Geometry: final body of the model. Coordinates: model frame, mm. A direction names the side the tool comes from. Round coordinates to 2 decimals unless told otherwise and drop trailing zeros. Loops run counter-clockwise (first coordinate to the right, second up) from the corner with the lowest first, then second, coordinate; pieces in that order, holes last. Notation, with made-up numbers: (13.5, -5.75) - (61.5, -5.75) arc R22 ccw to (61.5, 19.25) - close; hole circle Ø3 at (73.25, -26.75). An arc over 180 degrees is marked (long way). Answer as a JSON object with one key per item and string values. Group by question number.
Item 1: Section A-A (x = 37.5). Return the cut outline in (y, z), plus the area to 3 significant figures.
Item 2: Reachability of faces 1 (the face through (-8, 26, 3)), 2 (the face through (26.77, 26.97, 37.03)), 3 (the face through (-21.291, 21.135, 37.028)) from +Z, -Z, +X, -X, +Y, -Y: full face, straight path, thin tool, end or side. Return the list, or none.
Item 3: Line query: line 1 (Y direction, x = 0, z = 36); line 2 (X direction, y = 0, z = 10.5); line 3 (Z direction, x = -21, y = 24.5). Output: solid intervals per line, ascending.
Item 4: Draft query along Y for faces 4 (the face through (23, 0, 22)), 5 (the face through (28, -21, 1)), 6 (the face through (-15, -15, 0)). Return one class per face: released by +Y, released by -Y, zero draft, split by the parting line, or undercut.
Item 5: Section B-B (z = 18). Return the cut outline in (x, y), plus the area to 3 significant figures.
Item 6: First-contact query: pin 1 (6 mm diameter, centred on x = 12.5, z = 34.5, fed in from -Y) (3 decimals); pin 2 (1.4 mm diameter, centred on x = -2, y = -23.5, fed in from -Z); pin 3 (4 mm diameter, centred on x = 0, y = 37.5, fed in from -Z); pin 4 (1 mm diameter, centred on x = 5, z = 12, fed in from +Y). Flat tips, straight axial feed; report the tip coordinate or a pass-through.
Item 7: Section D-D (z = 26.5). Return the cut outline in (x, y), plus the area to 3 significant figures.
```python
from build123d import *

# Parameters (mm, degrees)
SKETCH_1_R               = 25
SKETCH_1_R_2             = 21
EXTRUDE_1_DEPTH          = 39
EXTRUDE_START            = -4
SKETCH_2_R               = 42.5
SKETCH_2_R_2             = 21
EXTRUDE_2_DEPTH          = 4
SKETCH_3_R               = 2.5
CUT_EXTRUDE_1_DEPTH      = 4
SKETCH_4_R               = 35
SKETCH_4_R_2             = 21
EXTRUDE_3_DEPTH          = 3
SKETCH_5_R               = 2
CUT_EXTRUDE_2_DEPTH      = 3
FILLET_1_R               = 2
CUT_EXTRUDE_3_DEPTH      = 42
PATTERN_CIRCULAR_1_COUNT = 4
CUT_EXTRUDE_4_DEPTH      = 5


with BuildPart() as part:
    # 草图1 → 凸台-拉伸1 (new body)
    with BuildSketch(Plane.XY):
        Circle(SKETCH_1_R)
        Circle(SKETCH_1_R_2, mode=Mode.SUBTRACT)
    extrude(amount=EXTRUDE_1_DEPTH)

    # 草图2 → 凸台-拉伸2 (add)
    with BuildSketch(Plane.XY.offset(39).offset(EXTRUDE_START)):
        Circle(SKETCH_2_R)
        Circle(SKETCH_2_R_2, mode=Mode.SUBTRACT)
    extrude(amount=EXTRUDE_2_DEPTH)

    # 草图3 → 切除-拉伸1 (cut)
    with BuildSketch(Plane.XY.offset(39)):
        with Locations((0, 37.5)):
            Circle(SKETCH_3_R)
        with Locations((37.5, 0)):
            Circle(SKETCH_3_R)
        with Locations((0, -37.5)):
            Circle(SKETCH_3_R)
        with Locations((-37.5, 0)):
            Circle(SKETCH_3_R)
    extrude(amount=-CUT_EXTRUDE_1_DEPTH, mode=Mode.SUBTRACT)

    # 草图4 → 凸台-拉伸3 (add)
    with BuildSketch(Plane(origin=(0, 0, 0), x_dir=(-1, 0, 0), z_dir=(0, 0, -1))):
        Circle(SKETCH_4_R)
        with Locations(Location((0, 0, 0), (0, 0, 180))):
            Circle(SKETCH_4_R_2, mode=Mode.SUBTRACT)
    extrude(amount=-EXTRUDE_3_DEPTH)

    # 草图5 → 切除-拉伸2 (cut)
    with BuildSketch(Plane(origin=(0, 0, 0), x_dir=(-1, 0, 0), z_dir=(0, 0, -1))):
        with Locations((0, 30)):
            Circle(SKETCH_5_R)
        with Locations((30, 0)):
            Circle(SKETCH_5_R)
        with Locations((0, -30)):
            Circle(SKETCH_5_R)
        with Locations((-30, 0)):
            Circle(SKETCH_5_R)
    extrude(amount=-CUT_EXTRUDE_2_DEPTH, mode=Mode.SUBTRACT)

    # 圆角1
    fillet_1_edges = [part.edges().sort_by_distance(p)[0] for p in [
        (-25, 0, 35),
        (-25, 0, 3),
    ]]
    fillet(fillet_1_edges, radius=FILLET_1_R)

    # 草图6 → 切除-拉伸3 (cut)
    with BuildSketch(Plane(origin=(0, 0, 0), x_dir=(0, 0, -1), z_dir=(1, 0, 0))):
        Polygon((-13, 0), (-22, 5.196152423), (-22, -5.196152423), align=None)
    cut_extrude_3 = extrude(amount=-CUT_EXTRUDE_3_DEPTH, mode=Mode.SUBTRACT)

    # 阵列(圆周)1: 切除-拉伸3 ×4 about axis
    pattern_circular_1_axis = Axis((0, 0, 0), (0, 0, 1))
    for i in range(1, PATTERN_CIRCULAR_1_COUNT):
        add(cut_extrude_3.rotate(pattern_circular_1_axis, i * 360 / PATTERN_CIRCULAR_1_COUNT), mode=Mode.SUBTRACT)

    # 草图7 → 切除-拉伸4 (cut)
    with BuildSketch(Plane.XY.offset(39)):
        with BuildLine():
            ThreePointArc((-19, 32.908965344), (-26.870057685, 26.870057685), (-32.908965344, 19))
            ThreePointArc((-32.908965344, 19), (-31.444863729, 13.535898385), (-25.980762114, 15))
            ThreePointArc((-25.980762114, 15), (-21.213203436, 21.213203436), (-15, 25.980762114))
            ThreePointArc((-15, 25.980762114), (-13.535898385, 31.444863729), (-19, 32.908965344))
        make_face()
        with BuildLine():
            ThreePointArc((25.980762114, 15), (21.213203436, 21.213203436), (15, 25.980762114))
            ThreePointArc((15, 25.980762114), (13.535898385, 31.444863729), (19, 32.908965344))
            ThreePointArc((19, 32.908965344), (26.870057685, 26.870057685), (32.908965344, 19))
            ThreePointArc((32.908965344, 19), (31.444863729, 13.535898385), (25.980762114, 15))
        make_face()
        with BuildLine():
            ThreePointArc((15, -25.980762114), (21.213203436, -21.213203436), (25.980762114, -15))
            ThreePointArc((25.980762114, -15), (31.444863729, -13.535898385), (32.908965344, -19))
            ThreePointArc((32.908965344, -19), (26.870057685, -26.870057685), (19, -32.908965344))
            ThreePointArc((19, -32.908965344), (13.535898385, -31.444863729), (15, -25.980762114))
        make_face()
        with BuildLine():
            ThreePointArc((-25.980762114, -15), (-21.213203436, -21.213203436), (-15, -25.980762114))
            ThreePointArc((-15, -25.980762114), (-13.535898385, -31.444863729), (-19, -32.908965344))
            ThreePointArc((-19, -32.908965344), (-26.870057685, -26.870057685), (-32.908965344, -19))
            ThreePointArc((-32.908965344, -19), (-31.444863729, -13.535898385), (-25.980762114, -15))
        make_face()
    extrude(amount=-CUT_EXTRUDE_4_DEPTH, mode=Mode.SUBTRACT)


solid = part.part
```
Values:
{
 "1": {"outline": "(-20, 35) - (-2.5, 35) - (-2.5, 39) - (-20, 39) - close; (2.5, 35) - (20, 35) - (20, 39) - (2.5, 39) - close", "area": "140 mm^2"},
 "2": {"face 1": "none", "face 2": "+Z, -Z", "face 3": "+Z"},
 "3": {"line 1": "y = -42.5 to -40, -35 to -21, 21 to 35, 40 to 42.5", "line 2": "x = -25 to -21, 21 to 25", "line 3": "z = 0 to 3"},
 "4": {"face 4": "undercut", "face 5": "split by the parting line", "face 6": "zero draft"},
 "5": {"outline": "(-24.83, -2.89) arc R25 ccw to (-2.89, -24.83) - (-2.89, -20.8) arc R21 cw to (-20.8, -2.89) - close; (-24.83, 2.89) - (-20.8, 2.89) arc R21 cw to (-2.89, 20.8) - (-2.89, 24.83) arc R25 ccw to start; (2.89, -24.83) arc R25 ccw to (24.83, -2.89) - (20.8, -2.89) arc R21 cw to (2.89, -20.8) - close; (2.89, 20.8) arc R21 cw to (20.8, 2.89) - (24.83, 2.89) arc R25 ccw to (2.89, 24.83) - close", "area": "485 mm^2"},
 "6": {"pin 1": "stops at y = -41.415", "pin 2": "stops at z = 0", "pin 3": "passes through", "pin 4": "stops at y = 24.59"},
 "7": {"outline": "circle Ø50 at (0, 0); hole circle Ø42 at (0, 0)", "area": "578 mm^2"}
}
